Input: dimensioned drawing with shaded views. Units: mm. Origin: part minimum x, y, z. A direction names the side the tool comes from. Coordinates: 2 decimals unless noted, no trailing zeros. Order: outer loops, then holes, each group sorted by start corner. A loop starts at its lowest first (then second) coordinate and runs counter-clockwise, first axis right, second up. Notation, with made-up numbers: M 15,78 L 29,78 A22 ccw 29,89 Z; hole C 42.25,-31.75 d3. An arc over 180 degrees is marked long. Write item = value, one per line.
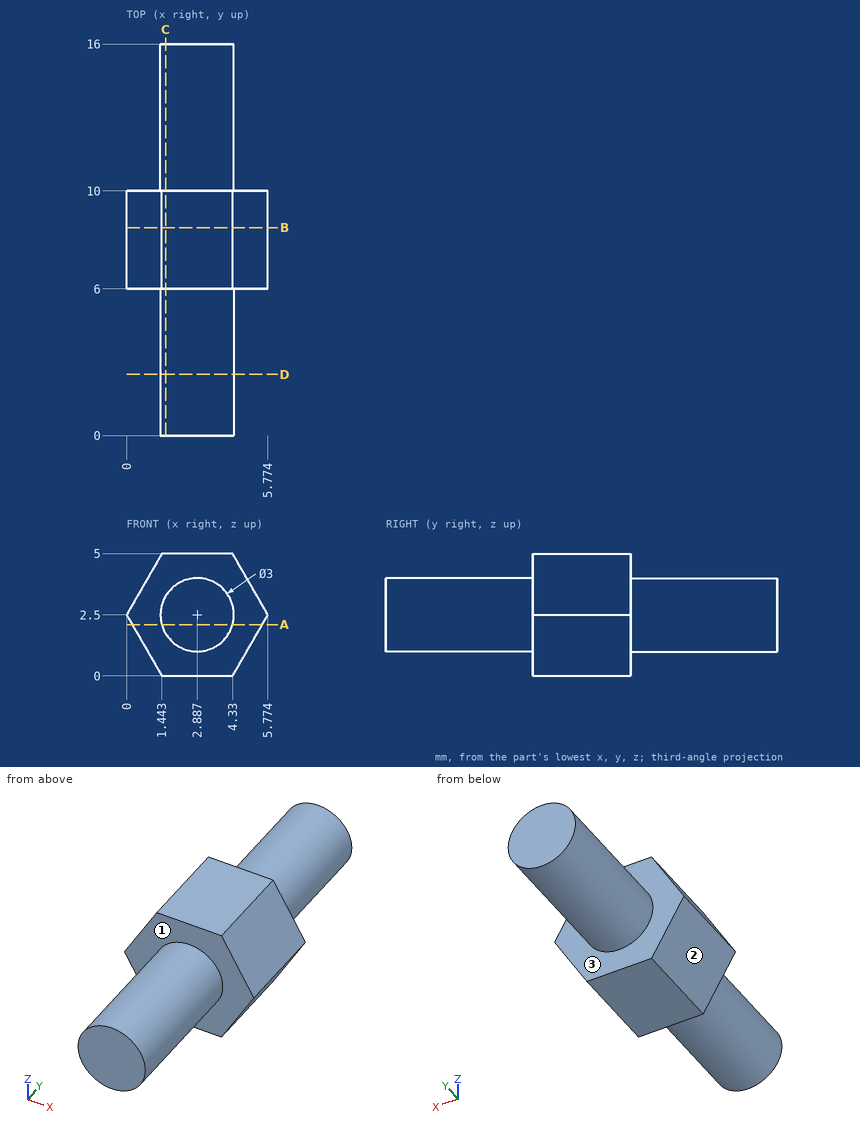
1) Section A-A, the plane z = 2.1. Return loops of the section in (x, y).
Numbers:
outline = M 0.23,6 L 1.44,6 L 1.44,0 L 4.33,0 L 4.33,6 L 5.54,6 L 5.54,10 L 4.33,10 L 4.33,16 L 1.44,16 L 1.44,10 L 0.23,10 Z
2) Section B-B, the plane y = 8.5. Return loops of the section in (x, z).
Numbers:
outline = M 0,2.5 L 1.44,0 L 4.33,0 L 5.77,2.5 L 4.33,5 L 1.44,5 Z
3) Line query: L1, parallel to Y at x = 1.15, z = 1.7; L2, parallel to X at y = 7.75, z = 3.55 (1 decimal); L3, parallel to X at y = 8, z = 1.75. Output: solid intervals per line, ascending.
Numbers:
L1 = 6 to 10
L2 = 0.6 to 5.2
L3 = 0.43 to 5.34
4) Section D-D, the plane y = 2.5. Return loops of the section in (x, z).
Numbers:
outline = C 2.89,2.5 d3
5) Pin query (flat end, axial travel): pin 1 (2 mm diameter, centred on x = 1, z = 3, fed in from +Y); pin 2 (1 mm diameter, centred on x = 2.5, y = 12, fed in from +Z); pin 3 (1.5 mm diameter, centred on y = 14, z = 3, fed in from +X). Return the tip coordinate at first contact, or that it passes through.
Numbers:
pin_1 = 16
pin_2 = 4
pin_3 = 4.39
6) Section C-C, the plane x = 1.6. Return loops of the section in (y, z).
Numbers:
outline = M 0,1.73 L 6,1.73 L 6,0 L 10,0 L 10,1.73 L 16,1.73 L 16,3.27 L 10,3.27 L 10,5 L 6,5 L 6,3.27 L 0,3.27 Z
7) Set-up query: the marked faces 1, 2 and 3. Return all of +Z, -Z, +X, -X, +Y, -Y with unobstructed straight access to the full face (end or side cutting, diameter ignored); none if empty.
Numbers:
face_1 = -Y
face_2 = -Z, -X, +Y, -Y
face_3 = +Y
